from build123d import *

# Parameters (mm, degrees)
F1_DEPTH = 19.05
F3_DEPTH = 12.7
F4_R     = 25.4
F5_R     = 25.4
F6_R     = 25.4
F7_R     = 25.4


with BuildPart() as f1:
    # F0 (on Front) → F1 (new body)
    with BuildSketch(Plane.XZ):
        Polygon((165.1, 163.4293), (0, 163.4293), (-165.1, 163.4293), (-165.1, -141.3707), (165.1, -141.3707), align=None)
    extrude(amount=F1_DEPTH)

    # F2 (on Front) → F3 (cut)
    with BuildSketch(Plane.XZ):
        Polygon((143.880641, -106.450708), (143.880641, 13.691292), (143.880641, 133.833292), (124.830641, 133.833292), (124.830641, 23.343292), (124.830641, 13.691292), (124.830641, 4.039292), (124.830641, -106.450708), align=None)
        Polygon((124.830641, 13.691292), (124.830641, 23.343292), (-124.830641, 23.343292), (-124.830641, 13.691292), (-124.830641, 4.039292), (124.830641, 4.039292), align=None)
        Polygon((-124.830641, 13.691292), (-124.830641, 23.343292), (-124.830641, 133.833292), (-143.880641, 133.833292), (-143.880641, 13.691292), (-143.880641, -106.450708), (-124.830641, -106.450708), (-124.830641, 4.039292), align=None)
    extrude(amount=F3_DEPTH, mode=Mode.SUBTRACT)

    # F4
    f4_edges = [f1.edges().sort_by_distance(p)[0] for p in [
        (165.1, -9.525, 163.4293),
    ]]
    fillet(f4_edges, radius=F4_R)

    # F5
    f5_edges = [f1.edges().sort_by_distance(p)[0] for p in [
        (165.1, -9.525, -141.3707),
    ]]
    fillet(f5_edges, radius=F5_R)

    # F6
    f6_edges = [f1.edges().sort_by_distance(p)[0] for p in [
        (-165.1, -9.525, -141.3707),
    ]]
    fillet(f6_edges, radius=F6_R)

    # F7
    f7_edges = [f1.edges().sort_by_distance(p)[0] for p in [
        (-165.1, -9.525, 163.4293),
    ]]
    fillet(f7_edges, radius=F7_R)


solid = f1.part
Build history of the part. All positions in model axes, mm. A direction names the side the tool comes from. Round coordinates to 2 decimals unless told otherwise and drop trailing zeros. Write each loop counter-clockwise with the first axis right and the second up, starting at its lowest first coordinate (ties: lowest second). Pieces come first, ordered by that corner, then holes. Notation, with made-up numbers: (9, -16) -> (48, -16) arc R24 ccw to (48, 23) -> close; hole circle Ø9 at (-33, 53). An arc over 180 degrees is marked (long way). Use one line per item in the form item = value.
Q1. Band-saw the part on D-D, the plane x = 16. Write the cut outline in (y, z), then the cut area to 3 significant figures.
Conclusion:
outline = (-19.05, -141.37) -> (0, -141.37) -> (0, 4.04) -> (-12.7, 4.04) -> (-12.7, 23.34) -> (0, 23.34) -> (0, 163.43) -> (-19.05, 163.43) -> close
area = 5,560 mm²
Q2. Band-saw the part on A-A, the plane y = -5.5. Write the cut outline in (x, z), then the cut area to 3 significant figures.
Conclusion:
outline = (-165.1, -115.97) arc R25.4 ccw to (-139.7, -141.37) -> (139.7, -141.37) arc R25.4 ccw to (165.1, -115.97) -> (165.1, 138.03) arc R25.4 ccw to (139.7, 163.43) -> (-139.7, 163.43) arc R25.4 ccw to (-165.1, 138.03) -> close; hole (-143.88, -106.45) -> (-124.83, -106.45) -> (-124.83, 4.04) -> (124.83, 4.04) -> (124.83, -106.45) -> (143.88, -106.45) -> (143.88, 133.83) -> (124.83, 133.83) -> (124.83, 23.34) -> (-124.83, 23.34) -> (-124.83, 133.83) -> (-143.88, 133.83) -> close
area = 86,100 mm²
Q3. Two-plate mould, pull along Z, no slides. Class faces 3 (the flat face through (-2, -9, -141.371)), 4 (the flat face through (-1, -12.7, 14)), 5 (the flat face through (165.1, -9, 9)): released by +Z, released by -Z, zero draft, split by the parting line, or undercut.
Conclusion:
face_3 = released by -Z
face_4 = undercut
face_5 = zero draft
Q4. Drill centre lines: L1, parallel to X at y = -9.25, z = -24; L2, parallel to Z at x = 51, y = -11; L3, parallel to Z at x = -137, y = -4.25. Where is each one in solid material? Low to high.
Conclusion:
L1 = -165.1 to -143.88, -124.83 to 124.83, 143.88 to 165.1
L2 = -141.37 to 4.04, 23.34 to 163.43
L3 = -141.37 to -106.45, 133.83 to 163.43
Q5. Band-saw the part on B-B, the plane x = -128.5. Write the cut outline in (y, z), then the cut area to 3 significant figures.
Conclusion:
outline = (-19.05, -141.37) -> (0, -141.37) -> (0, -106.45) -> (-12.7, -106.45) -> (-12.7, 133.83) -> (0, 133.83) -> (0, 163.43) -> (-19.05, 163.43) -> close
area = 2,750 mm²
Q6. Tool access for faces 1 (the flat face through (-2, -19.05, 13)), 2 (the flat face through (134, -6, -106.451)): list every direction of +Z, -Z, +X, -X, +Y, -Y with a clear straight run to the whole face (end or side of a thin tool).
Conclusion:
face_1 = +Z, -Z, +X, -X, -Y
face_2 = +Y
Q7. Band-saw the part on C-C, the plane z = 112. Write the cut outline in (x, y), then the cut area to 3 significant figures.
Conclusion:
outline = (-165.1, -19.05) -> (165.1, -19.05) -> (165.1, 0) -> (143.88, 0) -> (143.88, -12.7) -> (124.83, -12.7) -> (124.83, 0) -> (-124.83, 0) -> (-124.83, -12.7) -> (-143.88, -12.7) -> (-143.88, 0) -> (-165.1, 0) -> close
area = 5,810 mm²
